For this review, take the finished solid that the model builds, in its own axes (mm). Face numbers are marked on the shaded views. A direction names the side the tool comes from. Round coordinates to 2 decimals unless told otherwise and drop trailing zeros. Order: outer loops, then holes, each group sorted by start corner. A loop starts at its lowest first (then second) coordinate and runs counter-clockwise, first axis right, second up. Notation, with made-up numbers: M 12,-8.5 L 33,-8.5 A20 ccw 33,24.5 Z; hole C -35,15 d4. An arc over 180 degrees is marked long. Put each result on its own line as item: value.
from build123d import *

# Parameters (mm, degrees)
CROQUIS1_R              = 3
SALIENTE_EXTRUIR1_DEPTH = 4.5
CROQUIS2_R              = 3.5
SALIENTE_EXTRUIR2_DEPTH = 10.55
CROQUIS3_W              = 7
CROQUIS3_H              = 7
SALIENTE_EXTRUIR3_DEPTH = 18
CROQUIS4_R              = 3.5
SALIENTE_EXTRUIR4_DEPTH = 10.55
CROQUIS5_R              = 3
SALIENTE_EXTRUIR5_DEPTH = 4.5
CROQUIS6_R              = 1.25
CORTAR_EXTRUIR1_DEPTH   = 8
CHAFL_N1_SIZE           = 1.5


with BuildPart() as part:
    # Croquis1 → Saliente-Extruir1 (new body)
    with BuildSketch(Plane.XY):
        Circle(CROQUIS1_R)
    extrude(amount=SALIENTE_EXTRUIR1_DEPTH)

    # Croquis2 → Saliente-Extruir2 (add)
    with BuildSketch(Plane.XY.offset(4.5)):
        Circle(CROQUIS2_R)
    extrude(amount=SALIENTE_EXTRUIR2_DEPTH)

    # Croquis3 → Saliente-Extruir3 (add)
    with BuildSketch(Plane.XY.offset(15.05)):
        Rectangle(CROQUIS3_W, CROQUIS3_H)
    extrude(amount=SALIENTE_EXTRUIR3_DEPTH)

    # Croquis4 → Saliente-Extruir4 (add)
    with BuildSketch(Plane.XY.offset(33.05)):
        Circle(CROQUIS4_R)
    extrude(amount=SALIENTE_EXTRUIR4_DEPTH)

    # Croquis5 → Saliente-Extruir5 (add)
    with BuildSketch(Plane.XY.offset(43.6)):
        Circle(CROQUIS5_R)
    extrude(amount=SALIENTE_EXTRUIR5_DEPTH)

    # Croquis6 → Cortar-Extruir1 (cut, through all)
    with BuildSketch(Plane(origin=(0, 3.5, 0), x_dir=(1, 0, 0), z_dir=(0, 1, 0))):
        with Locations((0, -24.05)):
            Circle(CROQUIS6_R)
    extrude(amount=-CORTAR_EXTRUIR1_DEPTH, mode=Mode.SUBTRACT)

    # Chaflán1
    chafl_n1_edges = [part.edges().sort_by_distance(p)[0] for p in [
        (3.5, -3.5, 24.05),
        (3.5, 3.5, 24.05),
        (-3.5, 3.5, 24.05),
        (-3.5, -3.5, 24.05),
    ]]
    chamfer(chafl_n1_edges, length=CHAFL_N1_SIZE)


solid = part.part
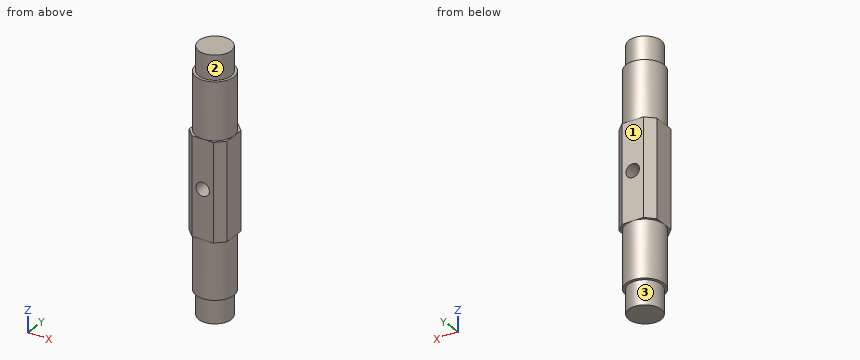
(1) For the marked faces 1, 2 and 3, list the 3-axis set-ups (+Z, -Z, +X, -X, +Y, -Y) from which the entire face can be reached by the end or side of a thin tool; tool diameter is ignored.
A:
face 1: +Z, -Z, +X, -X, +Y
face 2: +Z
face 3: -Z
(2) To check wall thickness, follow L1, parallel to Z at x = 0, y = 2.25; L2, parallel to X at y = 1.5, z = 24.05; L3, parallel to Z at x = 0.5, y = 1.5. State the ranges of each line that lie inside material, in increasing order.
A:
L1: z = 0 to 22.8, 25.3 to 48.1
L2: x = -3.5 to -1.25, 1.25 to 3.5
L3: z = 0 to 22.9, 25.2 to 48.1
(3) Add section A-A on z = 24.05. Give the boundary of the cut face in (x, y).
A:
outline: M -3.5,-2 L -2,-3.5 L -1.25,-3.5 L -1.25,3.5 L -2,3.5 L -3.5,2 Z; M 1.25,-3.5 L 2,-3.5 L 3.5,-2 L 3.5,2 L 2,3.5 L 1.25,3.5 Z
(4) Add section D-D on x = -2.5. Give the boundary of the cut face in (y, z), then the cut area to 3 significant figures.
A:
outline: M -3,15.05 L -2.45,15.05 L -2.45,4.5 L -1.66,4.5 L -1.66,0 L 1.66,0 L 1.66,4.5 L 2.45,4.5 L 2.45,15.05 L 3,15.05 L 3,33.05 L 2.45,33.05 L 2.45,43.6 L 1.66,43.6 L 1.66,48.1 L -1.66,48.1 L -1.66,43.6 L -2.45,43.6 L -2.45,33.05 L -3,33.05 Z
area: 241 mm2
(5) Add section C-C on y = 1.5. Give the boundary of the cut face in (x, z).
A:
outline: M -3.5,15.05 L -3.16,15.05 L -3.16,4.5 L -2.6,4.5 L -2.6,0 L 2.6,0 L 2.6,4.5 L 3.16,4.5 L 3.16,15.05 L 3.5,15.05 L 3.5,33.05 L 3.16,33.05 L 3.16,43.6 L 2.6,43.6 L 2.6,48.1 L -2.6,48.1 L -2.6,43.6 L -3.16,43.6 L -3.16,33.05 L -3.5,33.05 Z; hole C 0,24.05 d2.5
(6) Insertion check: pin 1 Ø4 at (y, z) = (2.5, 7.5) entering from +X; pin 2 Ø4 at (x, z) = (2.5, 41) entering from -Y. Each pin has a flat end and moves straight along its axis. Give the tip position at first contact, or say it passes through.
A:
pin 1: stops at x = 3.46
pin 2: stops at y = -3.46
(7) Add section B-B on x = 0.75. Give the boundary of the cut face in (y, z), then the cut area to 3 significant figures.
A:
outline: M -3.5,15.05 L -3.42,15.05 L -3.42,4.5 L -2.9,4.5 L -2.9,0 L 2.9,0 L 2.9,4.5 L 3.42,4.5 L 3.42,15.05 L 3.5,15.05 L 3.5,23.05 L -3.5,23.05 Z; M -3.5,25.05 L 3.5,25.05 L 3.5,33.05 L 3.42,33.05 L 3.42,43.6 L 2.9,43.6 L 2.9,48.1 L -2.9,48.1 L -2.9,43.6 L -3.42,43.6 L -3.42,33.05 L -3.5,33.05 Z
area: 309 mm2
